from build123d import *

# Parameters (mm, degrees)
SKETCH_1_R      = 18.5
SKETCH_1_R_2    = 1.6
EXTRUDE_1_DEPTH = 3.8
CHAMFER_1_SIZE  = 1


with BuildPart() as part:
    # Эскиз1 → Бобышка-Вытянуть1 (new body)
    with BuildSketch(Plane(origin=(0, 0, 0), x_dir=(1, 0, 0), z_dir=(0, 1, 0))):
        Circle(SKETCH_1_R)
        with Locations((-13.423393759, -7.75)):
            Circle(SKETCH_1_R_2, mode=Mode.SUBTRACT)
        with Locations((0, -15.5)):
            Circle(SKETCH_1_R_2, mode=Mode.SUBTRACT)
        with Locations((-13.423393759, 7.75)):
            Circle(SKETCH_1_R_2, mode=Mode.SUBTRACT)
        with Locations((0, 15.5)):
            Circle(SKETCH_1_R_2, mode=Mode.SUBTRACT)
        with Locations((13.423393759, 7.75)):
            Circle(SKETCH_1_R_2, mode=Mode.SUBTRACT)
        with Locations((13.423393759, -7.75)):
            Circle(SKETCH_1_R_2, mode=Mode.SUBTRACT)
        with BuildLine():
            ThreePointArc((10.767857143, -5.296532125), (13.5, 0), (10.767857143, 5.296532125))
            ThreePointArc((10.767857143, 5.296532125), (-12, 0), (10.767857143, -5.296532125))
        make_face(mode=Mode.SUBTRACT)
    extrude(amount=EXTRUDE_1_DEPTH)

    # Фаска1
    chamfer_1_edges = [part.edges().sort_by_distance(p)[0] for p in [
        (-18.5, 0, 0),
    ]]
    chamfer(chamfer_1_edges, length=CHAMFER_1_SIZE)


solid = part.part
Work out the finished part from the listing and answer in its coordinate system (mm). Round coordinates to 2 decimals unless told otherwise and drop trailing zeros. Order: outer loops, then holes, each group sorted by start corner. A loop starts at its lowest first (then second) coordinate and runs counter-clockwise, first axis right, second up. Notation, with made-up numbers: M -40,19 L -27,19 A23 cw -27,44 Z; hole C 45,50.25 d4. An arc over 180 degrees is marked long. Put each result on its own line as item: value. Start each with the question number.
Q1. Section C-C, the plane z = 8.5 is taken. Give the number of separate pieces and of enclosed holes in the cut face, and give its area (3 significant figures).
Q2. For a pull along X with two mould halves and no side action, classify faces 1 (the cylindrical face through (13.5, 1.9, 0.1)), 2 (the cylindrical face through (-4.01, 2.38, 18.06)), 3 (the cylindrical face through (12.15, 1.87, 8.72)), 4 (the flat face through (-12, 0, 3)) as pulls with the +X half, pulls with the -X half, needs draft (parallel to the pull), parting line crosses it, or undercut.
Q3. Section B-B, the plane x = 0 is taken. Write down the section's boundary in (y, z), and give its area (3 significant figures).
Q4. Flat-ended cylindrical pins translate along their axes: pin 1 (2 mm diameter, centred on x = 3, y = 1.5, fed in from -Z); pin 2 (3 mm diameter, centred on x = -13.42, z = -7.75, fed in from +Y); pin 3 (1.5 mm diameter, centred on x = -11.5, y = 2, fed in from -Z); pin 4 (1.5 mm diameter, centred on x = -8.5, y = 3, fed in from +Z). Find the tip coordinate at first contact, or state that the pin passes through.
Q5. Section A-A, the plane y = 1.5 is taken. Write down the section's boundary in (x, z), and give its area (3 significant figures).
Q6. Straight lines are drawn through the part: L1, parallel to X at y = 1.65, z = 7.75; L2, parallel to Z at x = 0.5, y = 1.3; L3, parallel to X at y = 1.25, z = -7.5. For each, find the intervals that lie inside material, in ascending order. Write a range as [from, to].
Findings below:
1. separate pieces: 4
1. enclosed holes: 0
1. area: 37.9 mm^2
2. face 1: undercut
2. face 2: parting line crosses it
2. face 3: undercut
2. face 4: needs draft
3. outline: M 0,-17.5 L 1,-18.5 L 3.8,-18.5 L 3.8,-17.1 L 0,-17.1 Z; M 0,-13.9 L 3.8,-13.9 L 3.8,-12 L 0,-12 Z; M 0,12 L 3.8,12 L 3.8,13.9 L 0,13.9 Z; M 0,17.1 L 3.8,17.1 L 3.8,18.5 L 1,18.5 L 0,17.5 Z
3. area: 24.1 mm^2
4. pin 1: stops at z = -18.39
4. pin 2: passes through
4. pin 3: stops at z = -15.06
4. pin 4: stops at z = 16.8
5. outline: C 0,0 d37; hole C -13.42,-7.75 d3.2; hole C -13.42,7.75 d3.2; hole C 0,-15.5 d3.2; hole C 0,15.5 d3.2; hole M 10.77,-5.3 A6.5 ccw 10.77,5.3 A12 ccw long Z; hole C 13.42,-7.75 d3.2; hole C 13.42,7.75 d3.2
5. area: 563 mm^2
6. L1: x = [-16.8, -15.02], [-11.82, -9.16], [9.16, 11.82], [15.02, 16.8]
6. L2: z = [-18.49, -17.02], [-13.98, -11.99], [11.99, 13.98], [17.02, 18.49]
6. L3: x = [-16.91, -15], [-11.84, -9.37], [9.37, 11.84], [15, 16.91]
